Check sheet for the modelled part. Datum: model origin and axes. Units: mm. Face numbers are marked on the shaded views. A direction names the side the tool comes from. Coordinates: 2 decimals unless noted, no trailing zeros. Order: outer loops, then holes, each group sorted by start corner. A loop starts at its lowest first (then second) coordinate and runs counter-clockwise, first axis right, second up. Notation, with made-up numbers: (-10, 14) -> (10, 14) arc R32 cw to (10, 41) -> close; hole circle Ø5 at (6, 50.25). An arc over 180 degrees is marked (long way). Put each result on its own line as item: value. Start each with the question number.
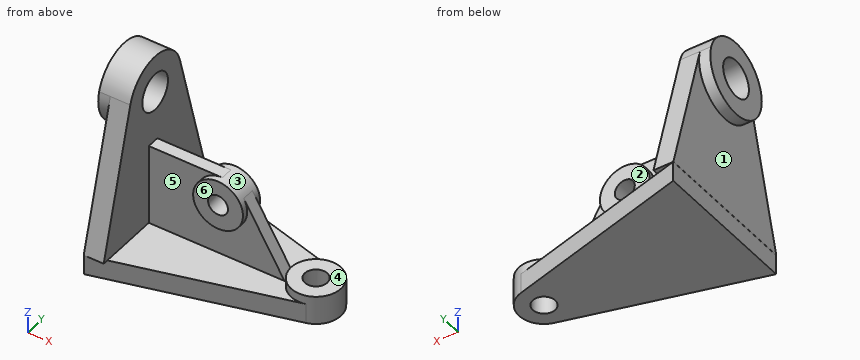
Autodesk Fusion 360 part; units mm, degrees
sketch "Sketch1" plane through (0, 0, 0) normal (0, 0, 1) x (1, 0, 0)
  line L0 (0.1058, -52.6202) -> (0.1058, 67.3798)
  line L1 (0.1058, 67.3798) -> (0.1058, 7.3798)
  circle A0 centre (145.1058, 7.3798) radius 9
  circle A1 centre (145.1058, 7.3798) radius 20
  line L2 (0.1058, 67.3798) -> (150.3351, 26.684)
  line L3 (0.1058, -52.6202) -> (150.3351, -11.9245)
  dimension "d1" = 120
  dimension "d2" = 60
  dimension "d3" = 145
  dimension "d4" = 18
  dimension "d5" = 40
extrude "Extrude1" add sketch "Sketch1" along normal blind 16 contours L0 L1 A1 L2 L3
extrude "Extrude2" add sketch "Sketch1" along normal blind 23 contours A1
sketch "Sketch2" plane through (0, 0, 16) normal (0, 0, 1) x (-1, 0, 0)
  line L0 (-0.1058, -67.3798) -> (-0.1058, 52.6202)
  line L1 (-0.1058, 52.6202) -> (-150.3351, 11.9245)
  arc A0 (-150.3351, -26.684) -> (-150.3351, 11.9245) centre (-145.1058, -7.3798) ccw
  line L2 (-150.3351, -26.684) -> (-0.1058, -67.3798)
sketch "Sketch3" plane through (0, 0, 0) normal (1, 0, 0) x (0, 1, 0)
sketch "Sketch4" plane through (0, 0, 0) normal (1, 0, 0) x (0, 1, 0)
  line L0 (-52.6, 16) -> (67.3803, 16)
  line L1 (67.3803, 16) -> (7.3902, 16)
  line L2 (7.3902, 16) -> (7.3902, 122)
  circle A0 centre (7.3902, 122) radius 30
  circle A1 centre (7.3902, 122) radius 15
  line L3 (-52.6, 16) -> (-21.5537, 129.8901)
  line L4 (67.3803, 16) -> (36.334, 129.8901)
  dimension "d10" = 106
  dimension "d11" = 60
  dimension "d12" = 30
extrude "Extrude3" add sketch "Sketch4" along normal blind 16 contours L0 L2 A0 L3 | L0 L1 L2 A0 L4
sketch "Sketch5" plane through (16, 0, 0) normal (1, 0, 0) x (0, 1, 0)
  line L0 (-52.6, 16) -> (-48.3146, 16)
  line L1 (-48.3146, 16) -> (63.0742, 16)
  line L2 (63.0742, 16) -> (67.3803, 16)
  line L3 (67.3803, 16) -> (36.334, 129.8901)
  arc A0 (-21.5537, 129.8901) -> (36.334, 129.8901) centre (7.3902, 122) ccw
  line L4 (-21.5537, 129.8901) -> (-52.6, 16)
  circle A1 centre (7.3902, 122) radius 15
  circle A2 centre (7.3902, 122) radius 30
  dimension "d15" = 30
  dimension "d16" = 60
extrude "Extrude4" add sketch "Sketch5" against normal blind 25 contours A0 A2
sketch "Sketch6" plane through (0, 0, 0) normal (0, 1, 0) x (1, 0, 0)
  line L0 (0, 0) -> (0, -61)
  circle A0 centre (75, -61) radius 20
  circle A1 centre (75, -61) radius 8
  line L1 (75, -81) -> (16, -81)
  line L2 (124.9247, -16.1323) -> (92.1937, -71.2165)
  line L3 (16, -81) -> (16, -16)
  line L4 (16, -16) -> (124.9247, -16.1323)
  dimension "d19" = 61
  dimension "d20" = 75
  dimension "d21" = 40
  dimension "d22" = 16
sketch "Sketch7" plane through (16, 0, 0) normal (1, 0, 0) x (0, 1, 0)
  circle A0 centre (7.3902, 122) radius 15
  line L0 (-52.6, 16) -> (-48.3146, 16)
  line L1 (-48.3146, 16) -> (63.0742, 16)
  line L2 (63.0742, 16) -> (67.3803, 16)
  line L3 (67.3803, 16) -> (36.334, 129.8901)
  arc A1 (36.334, 129.8901) -> (-21.5537, 129.8901) centre (7.3902, 122) ccw
  line L4 (-21.5537, 129.8901) -> (-52.6, 16)
sketch "Sketch8" plane through (0, 0, 0) normal (0, 1, 0) x (1, 0, 0)
extrude "Extrude5" add sketch "Sketch6" along normal blind 10 contours A0 L1 L2 L3 L4
extrude "Extrude6" add sketch "Sketch6" along normal blind 15 contours A0
extrude "Extrude7" add sketch "Sketch6" against normal blind 5 contours A0
1) Scan lines: line 1 along X through (y, z) = (10.25, 61); line 2 along X through (y, z) = (6.5, 20); line 3 along Z through (x, y) = (29, 59). Record each from-to range of solid material in increasing order. Write a range as [from, to].
2) Sectioned sample at A-A (z = 125). Record the boundary of the cut face in (x, y), plus the area to 3 significant figures.
3) Sectioned sample at D-D (z = 28). Record the boundary of the cut face in (x, y), plus the area to 3 significant figures.
4) Gauge pin test, flat ends, axial feed: pin 1 (6 mm diameter, centred on y = -34, z = 77.5, fed in from -X); pin 2 (5 mm diameter, centred on x = 97, z = 46.5, fed in from -Y); pin 3 (8 mm diameter, centred on x = 29, y = -40, fed in from +Z); pin 4 (3.5 mm diameter, centred on x = 7.5, y = -49.5, fed in from -Z). Record the tip position at first contact, or that the pin passes through.
5) Sectioned sample at B-B (x = 140). Record the boundary of the cut face in (y, z).
6) Sectioned sample at C-C (y = 58). Record the boundary of the cut face in (x, z).
7) Mould release check, pull along X, two halves, no side actions. Record for the marked faces 1, 2 and 3: +X half, -X half, draft (parallel to the pull), parting line (faces both ways), or undercut.
8) Access from +Z, -Z, +X, -X, +Y, -Y to the whole of each face (thin tool, end or side, straight path). Record for the marked faces 4, 5 and 6.
Entries:
1. line 1: x = [0, 16], [55, 67], [83, 95]
1. line 2: x = [0, 122.63], [125.13, 136.15], [154.06, 165.09]
1. line 3: z = [0, 16]
2. outline: (-9, -22.46) -> (0, -22.46) -> (0, -22.89) -> (16, -22.89) -> (16, -7.31) -> (-9, -7.31) -> close; (-9, 22.09) -> (16, 22.09) -> (16, 37.67) -> (0, 37.67) -> (0, 37.24) -> (-9, 37.24) -> close
2. area: 771 mm2
3. outline: (0, -49.33) -> (16, -49.33) -> (16, 0) -> (117.87, 0) -> (117.87, 10) -> (16, 10) -> (16, 64.11) -> (0, 64.11) -> close
3. area: 2,830 mm2
4. pin 1: stops at x = 0
4. pin 2: stops at y = 0
4. pin 3: stops at z = 16
4. pin 4: stops at z = 0
5. outline: (-14.72, 0) -> (-0.03, 0) -> (-0.03, 23) -> (-11.96, 23) -> (-11.96, 16) -> (-14.72, 16) -> close; (14.79, 0) -> (29.48, 0) -> (29.48, 16) -> (26.72, 16) -> (26.72, 23) -> (14.79, 23) -> close
6. outline: (0, 16) -> (0.11, 16) -> (0.11, 0) -> (34.73, 0) -> (34.73, 16) -> (16, 16) -> (16, 50.41) -> (0, 50.41) -> close
7. face 1: -X half
7. face 2: draft
7. face 3: undercut
8. face 4: +Z, +X, +Y, -Y
8. face 5: -Y
8. face 6: +Z, +X, -Y
